Input: part model. Units: mm. Frame: model coordinates. Give positions to 0.01 mm unless a question says otherwise; leave off trailing zeros. Loops run counter-clockwise (first coordinate to the right, second up) from the corner with the lowest first, then second, coordinate; pieces in that order, holes last. Notation, with made-up numbers: (81, 77.25) - (88, 77.25) arc R10 cw to (88, 93.25) - close; hole circle Ø6 at (71.25, 49). An arc over 180 degrees is marked (long way). Answer as a JSON object with one key per item and string values.
from build123d import *

# Parameters (mm, degrees)
SKETCH1_R           = 1.45
SKETCH1_R_2         = 1.5
BOSS_EXTRUDE1_DEPTH = 1.5
FILLET1_R           = 10


with BuildPart() as part:
    # Sketch1 → Boss-Extrude1 (new, symmetric)
    with BuildSketch(Plane(origin=(0, 0, 0), x_dir=(0, 0, -1), z_dir=(1, 0, 0))):
        with BuildLine():
            Line((-110, 14), (-127.759109434, 6.974045822))
            ThreePointArc((-127.759109434, 6.974045822), (-132.233383985, -1.981957648), (-123.818844483, -7.406407472))
            Line((-123.818844483, -7.406407472), (-115, -6))
            Line((-115, -6), (-91, -4.5))
            Line((-91, -4.5), (-6, -4.5))
            ThreePointArc((-6, -4.5), (5.167384395, -5.435819948), (4.797838271, 5.764611689))
            Line((4.797838271, 5.764611689), (-7.5, 16))
            Line((-7.5, 16), (-110, 14))
        make_face()
        with Locations((-125, 0)):
            Circle(SKETCH1_R, mode=Mode.SUBTRACT)
        with Locations((-106.5, 5)):
            Circle(SKETCH1_R_2, mode=Mode.SUBTRACT)
        Polygon((-98.5, 3.5), (-98.5, 6.5), (-97, 8), (-33, 8), (-31.5, 6.5), (-31.5, 3.5), (-33, 2), (-97, 2), align=None, mode=Mode.SUBTRACT)
        with Locations((-23.5, 8.5)):
            Circle(SKETCH1_R_2, mode=Mode.SUBTRACT)
        Circle(SKETCH1_R, mode=Mode.SUBTRACT)
    extrude(amount=BOSS_EXTRUDE1_DEPTH, both=True)

    # Fillet1
    # the kernel refuses this fillet: 10 mm, written as the material it adds along each edge
    with BuildSketch(Plane(origin=(1.5, -4.5, 6), x_dir=(0, -0.6894794553430702, -0.7243052399781623), z_dir=(-1, 0, 0))) as fillet1_piece_1:
        with BuildLine():
            CenterArc((4.143912969, 9.861667083), FILLET1_R, 226.411082638, 34.04773237)
            Line((-2.750881584, 2.618614683), (0, 0))
            ThreePointArc((0, 0), (1.243173891, 0.103749688), (2.486347782, 0))
        make_face()
    extrude(amount=3)
    with BuildSketch(Plane(origin=(1.5, -4.5, 91), x_dir=(0, 0, -1), z_dir=(-1, 0, 0))) as fillet1_piece_2:
        with BuildLine():
            CenterArc((FILLET1_R * 0.0312195418814, FILLET1_R), FILLET1_R, 266.423665625, 3.576334375)
            Line((-FILLET1_R * 0.0311587442738, FILLET1_R * 0.00194742151711), (0, 0))
            Line((0, 0), (FILLET1_R * 0.0312195418814, 0))
        make_face()
    extrude(amount=3)
    with BuildSketch(Plane(origin=(-1.5, -6, 115), x_dir=(0, 0.06237828615518053, -0.9980525784828885), z_dir=(1, 0, 0))) as fillet1_piece_3:
        with BuildLine():
            CenterArc((FILLET1_R * 0.04790007143, -FILLET1_R), FILLET1_R, 90, 5.484751657)
            Line((-FILLET1_R * 0.0476807691396, -FILLET1_R * 0.00457832909063), (0, 0))
            Line((0, 0), (FILLET1_R * 0.04790007143, 0))
        make_face()
    extrude(amount=3)
    # the kernel refuses this fillet: 10 mm, written as the material it takes off along each edge
    with BuildSketch(Plane(origin=(-6.013343282, 14, 110), x_dir=(0, 0.019508481784595348, -0.99980969146056), z_dir=(1, 0, 0))) as fillet1_2_piece_1:
        with BuildLine():
            CenterArc((FILLET1_R * 0.180533731282, -FILLET1_R), FILLET1_R, 90, 20.467183595)
            Line((-FILLET1_R * 0.169137109533, -FILLET1_R * 0.063127381613), (0, 0))
            Line((0, 0), (FILLET1_R * 0.180533731282, 0))
        make_face()
    extrude(amount=12.026686564, mode=Mode.SUBTRACT)
    with BuildSketch(Plane(origin=(-10.819315302, 16, 7.5), x_dir=(0, -0.6397117694155324, -0.7686148919135308), z_dir=(1, 0, 0))) as fillet1_2_piece_2:
        with BuildLine():
            CenterArc((FILLET1_R * 0.372772612074, -FILLET1_R), FILLET1_R, 90, 40.88815481)
            Line((-FILLET1_R * 0.281811924347, -FILLET1_R * 0.244011187465), (0, 0))
            Line((0, 0), (FILLET1_R * 0.372772612074, 0))
        make_face()
    extrude(amount=21.638630604, mode=Mode.SUBTRACT)


solid = part.part
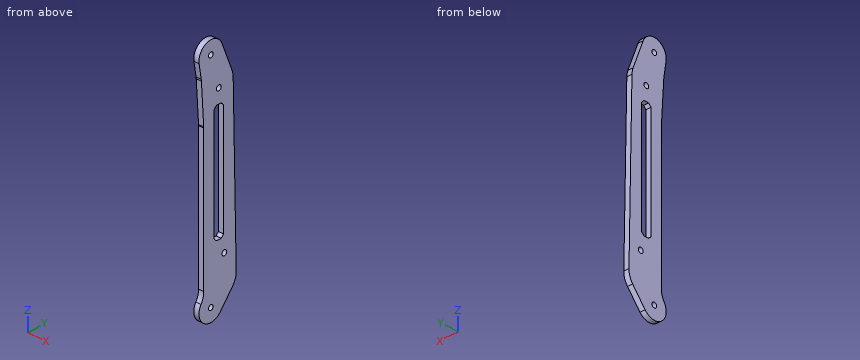
Item 1: Material intervals for line 1 (Z direction, x = -0.7, y = 4); line 2 (Z direction, x = -0.65, y = 1); line 3 (Y direction, x = -0.45, z = 82), sorted ascending. Write a range as [from, to].
Geometry check:
{"line 1": "z = [-6.34, 31.5], [98.5, 105.38], [107.62, 131.34]", "line 2": "z = [-7.43, -1.05], [1.05, 123.95], [126.05, 132.43]", "line 3": "y = [-4.5, 2], [8, 14.55]"}
Item 2: Cut plane A-A (x = -0.9). Return loops of the section in (y, z) (3 decimals), then the cut area to 3 significant figures.
Geometry check:
{"outline": "(-7.406, 123.819) - (-6.075, 115.473) arc R10 cw to (-5.97, 114.522) - (-4.519, 91.312) arc R10 cw to (-4.5, 90.688) - (-4.5, 9.798) arc R10 cw to (-6.214, 4.199) arc R7.5 ccw to (5.765, -4.798) - (13.615, 4.635) arc R10 ccw to (15.927, 11.227) - (14.035, 108.195) arc R10 ccw to (13.336, 111.679) - (6.974, 127.759) arc R7.5 ccw to start; hole circle Ø2.9 at (0, 0); hole circle Ø2.9 at (0, 125); hole (2, 33) - (3.5, 31.5) - (6.5, 31.5) - (8, 33) - (8, 97) - (6.5, 98.5) - (3.5, 98.5) - (2, 97) - close; hole circle Ø3 at (5, 106.5); hole circle Ø3 at (8.5, 23.5)", "area": "2,170 mm2"}
Item 3: Cut plane D-D (z = 27). Return loops of the section in (x, y), then the cut area to 3 significant figures.
Geometry check:
{"outline": "(-1.5, -4.5) - (1.5, -4.5) - (1.5, 15.62) - (-1.5, 15.62) - close", "area": "60.4 mm2"}
Item 4: Cut plane B-B (z = 106.5). Return loops of the section in (x, y), then the cut area to 3 significant figures.
Geometry check:
{"outline": "(-1.5, -5.47) - (1.5, -5.47) - (1.5, 3.5) - (-1.5, 3.5) - close; (-1.5, 6.5) - (1.5, 6.5) - (1.5, 14.07) - (-1.5, 14.07) - close", "area": "49.6 mm2"}
Item 5: Cut plane C-C (z = 125). Return loops of the section in (x, y).
Geometry check:
{"outline": "(-1.5, -7.5) - (1.5, -7.5) - (1.5, -1.45) - (-1.5, -1.45) - close; (-1.5, 1.45) - (1.5, 1.45) - (1.5, 8.07) - (-1.5, 8.07) - close"}
Item 6: Contact query for flat-ended pins moving along their axis: P1, Ø1.5, axis at x = 0, y = 5, coming from the +Z side; P2, Ø2.5, axis at y = 8.5, z = 23.5, coming from the -X side; P3, Ø1, axis at x = -1, z = 20, coming from the +Y side; P4, Ø0.9, axis at x = 0, z = 38.5, coming from the -Y side. Output: stop coordinate, or through.
Geometry check:
{"P1": "stops at z = 131.18", "P2": "passes through", "P3": "stops at y = 15.77", "P4": "stops at y = -4.5"}
